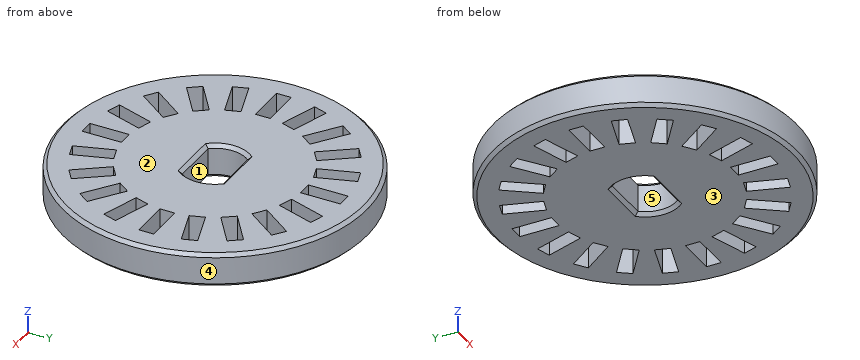
```python
from build123d import *

# Parameters (mm, degrees)
SKETCH002_R        = 13.4
PAD_DEPTH          = 3
POCKET_DEPTH       = 3.001
SKETCH003_W        = 1.3
SKETCH003_H        = 3.5
POCKET001_DEPTH    = 79.039937
POLARPATTERN_COUNT = 20
CHAMFER_SIZE       = 0.3
CHAMFER001_SIZE    = 0.3


with BuildPart() as part:
    # Sketch002 → Pad (new body)
    with BuildSketch(Plane.XY):
        Circle(SKETCH002_R)
    extrude(amount=PAD_DEPTH)

    # Sketch → Pocket (cut, through all)
    with BuildSketch(Plane.XY.offset(3)):
        with BuildLine():
            Line((-2.12132, 1.75), (2.12132, 1.75))
            ThreePointArc((2.12132, -1.75), (2.75, 0), (2.12132, 1.75))
            Line((-2.12132, -1.75), (2.12132, -1.75))
            ThreePointArc((-2.12132, 1.75), (-2.75, 0), (-2.12132, -1.75))
        make_face()
    extrude(amount=-POCKET_DEPTH, mode=Mode.SUBTRACT)

    # Sketch003 → Pocket001 (cut, through all)
    with BuildSketch(Plane.XY.offset(3)):
        with Locations((0, 9.65)):
            Rectangle(SKETCH003_W, SKETCH003_H)
    pocket001 = extrude(amount=-POCKET001_DEPTH, mode=Mode.SUBTRACT)

    # PolarPattern: Pocket001 ×20 about axis
    polarpattern_axis = Axis((0, 0, 3), (0, 0, 1))
    for i in range(1, POLARPATTERN_COUNT):
        add(pocket001.rotate(polarpattern_axis, i * 360 / POLARPATTERN_COUNT), mode=Mode.SUBTRACT)

    # Chamfer
    chamfer_edges = [part.edges().sort_by_distance(p)[0] for p in [
        (0, 1.75, 0),
        (2.75, 0, 0),
        (0, -1.75, 0),
        (-2.75, 0, 0),
        (2.75, 0, 3),
        (0, 1.75, 3),
        (-2.75, 0, 3),
        (0, -1.75, 3),
    ]]
    chamfer(chamfer_edges, length=CHAMFER_SIZE)

    # Chamfer001
    chamfer001_edges = [part.edges().sort_by_distance(p)[0] for p in [
        (-13.4, 0, 0),
        (-13.4, 0, 3),
    ]]
    chamfer(chamfer001_edges, length=CHAMFER001_SIZE)


solid = part.part
```
Check sheet for the modelled part. Datum: model origin and axes. Units: mm. Face numbers are marked on the shaded views. A direction names the side the tool comes from. Round coordinates to 2 decimals unless told otherwise and drop trailing zeros. Loops run counter-clockwise (first coordinate to the right, second up) from the corner with the lowest first, then second, coordinate; pieces in that order, holes last. Notation, with made-up numbers: (21.25, -22.5) - (69.25, -22.5) arc R13 cw to (69.25, -18.5) - close; hole circle Ø11 at (-32, 33). An arc over 180 degrees is marked (long way). Answer as a JSON object with one key per item and string values. Group by question number.
Q1. Set-up check for the marked faces 1 and 2: record each of +Z, -Z, +X, -X, +Y, -Y from which the full face is reachable in a straight line by a thin tool's end or side.
Q2. Gauge pin test, flat ends, axial feed: P1, Ø1.5, axis at y = -9.5, z = 1, coming from the +X side; P2, Ø3, axis at x = 9.5, y = -10, coming from the +Z side; P3, Ø0.9, axis at y = 9, z = 1, coming from the -X side; P4, Ø1.5, axis at x = 9.5, z = 1.5, coming from the -Y side. Record the tip position at first contact, or that the pin passes through.
Q3. Sectioned sample at B-B, the plane y = 0. Enter the section's corners in (x, z).
Q4. Scan lines: line 1 along Y through (x, z) = (-0.25, 2.35); line 2 along Y through (x, z) = (-9.5, 1.25); line 3 along X through (y, z) = (-3, 2.6). Record each from-to range of solid material in increasing order. Write a range as [from, to].
Q5. Sectioned sample at C-C, the plane z = 1.3. Count the separate pieces of the cut face and the enclosed holes in it, plus the area to 3 significant figures.
Q6. Mould release check, pull along Y, two halves, no side actions. Record for the marked faces 3, 4 and 5: released by +Y, released by -Y, zero draft, split by the parting line, or undercut.
Q7. Sectioned sample at A-A, the plane x = 0. Enter the section's corners in (y, z), plus the area to 3 significant figures.
Solution:
{
 "1": {"face 1": "+Z, -Z", "face 2": "+Z, +X, -X, +Y, -Y"},
 "2": {"P1": "stops at x = 10.15", "P2": "stops at z = 3", "P3": "stops at x = -10.32", "P4": "stops at y = -10.15"},
 "3": {"outline": "(-13.4, 0.3) - (-13.1, 0) - (-11.4, 0) - (-11.4, 3) - (-13.1, 3) - (-13.4, 2.7) - close; (-7.9, 0) - (-3.05, 0) - (-2.75, 0.3) - (-2.75, 2.7) - (-3.05, 3) - (-7.9, 3) - close; (2.75, 0.3) - (3.05, 0) - (7.9, 0) - (7.9, 3) - (3.05, 3) - (2.75, 2.7) - close; (11.4, 0) - (13.1, 0) - (13.4, 0.3) - (13.4, 2.7) - (13.1, 3) - (11.4, 3) - close"},
 "4": {"line 1": "y = [-13.4, -11.4], [-7.9, -1.75], [1.75, 7.9], [11.4, 13.4]", "line 2": "y = [-9.45, -6.32], [-6.1, -3.77], [-2.4, -0.65], [0.65, 2.4], [3.77, 6.1], [6.32, 9.45]", "line 3": "x = [-13.06, -11.01], [-7.33, 7.33], [11.01, 13.06]"},
 "5": {"separate pieces": "1", "enclosed holes": "21", "area": "455 mm²"},
 "6": {"face 3": "zero draft", "face 4": "split by the parting line", "face 5": "undercut"},
 "7": {"outline": "(-13.4, 0.3) - (-13.1, 0) - (-11.4, 0) - (-11.4, 3) - (-13.1, 3) - (-13.4, 2.7) - close; (-7.9, 0) - (-2.05, 0) - (-1.75, 0.3) - (-1.75, 2.7) - (-2.05, 3) - (-7.9, 3) - close; (1.75, 0.3) - (2.05, 0) - (7.9, 0) - (7.9, 3) - (2.05, 3) - (1.75, 2.7) - close; (11.4, 0) - (13.1, 0) - (13.4, 0.3) - (13.4, 2.7) - (13.1, 3) - (11.4, 3) - close", "area": "48.5 mm²"}
}
